Geometry: final body of the model. Coordinates: model frame, mm. A direction names the side the tool comes from. Give positions to 0.01 mm unless a question says otherwise; leave off trailing zeros. Order: outer loops, then holes, each group sorted by start corner. A loop starts at its lowest first (then second) coordinate and runs counter-clockwise, first axis right, second up. Notation, with made-up numbers: (36, -11.5) - (43, -11.5) arc R13 cw to (43, 11.5) - close; hole circle Ø9 at (86, -23.75). An arc over 180 degrees is marked (long way). One line per item, written item: value.
```python
from build123d import *

# Parameters (mm, degrees)
F1_DEPTH  = 6
F2_R      = 1.6
F2_W      = 10
F2_H      = 6
F2_W_2    = 6
F2_H_2    = 10
F3_DEPTH  = 6.001
F4_W      = 6
F4_H      = 10
F5_DEPTH  = 6.001
F7_DEPTH  = 6.001
F8_R      = 10
F9_R      = 8
F9_R_2    = 3
F9_R_3    = 1.5
F10_DEPTH = 6.001
F11_R     = 7.99999


# Not quite as in the source:
# - a fillet or chamfer is up to 0.001 mm smaller than in the source, because OpenCascade refuses the exact size


with BuildPart() as f1:
    # F0 (on Top) → F1 (new body)
    with BuildSketch(Plane.XY):
        Polygon((-150, -150), (150, -150), (150, -20.0961894323), (51.7949192431, 150), (-51.7949192431, 150), (-150, -20.0961894323), align=None)
    extrude(amount=F1_DEPTH)

    # F2 (on face) → F3 (cut, through all)
    with BuildSketch(Plane.XY.offset(6)):
        Polygon((-139.3974596216, -1.7320508076), (-142.3974596216, -6.9282032303), (-133.7372055837, -11.9282032303), (-130.7372055837, -6.7320508076), align=None)
        with Locations((-127.9070785648, -11.8301270189)):
            Circle(F2_R)
        Polygon((-50.7372055837, 131.8320137979), (-59.3974596216, 136.8320137979), (-62.3974596216, 131.6358613752), (-53.7372055837, 126.6358613752), align=None)
        with Locations((-47.9070785648, 126.7339375866)):
            Circle(F2_R)
        Polygon((133.7372055837, -11.9282032303), (142.3974596216, -6.9282032303), (139.3974596216, -1.7320508076), (130.7372055837, -6.7320508076), align=None)
        with Locations((127.9070785648, -11.8301270189)):
            Circle(F2_R)
        Polygon((53.7372055837, 126.6358613752), (62.3974596216, 131.6358613752), (59.3974596216, 136.8320137979), (50.7372055837, 131.8320137979), align=None)
        with Locations((47.9070785648, 126.7339375866)):
            Circle(F2_R)
        with Locations((-145, -35.0480947162)):
            Rectangle(F2_W, F2_H)
        with Locations((-135, -35.0480947162)):
            Circle(F2_R)
        with Locations((-145, -135.0480947162)):
            Rectangle(F2_W, F2_H)
        with Locations((-135, -135.0480947162)):
            Circle(F2_R)
        with Locations((145, -135.0480947162)):
            Rectangle(F2_W, F2_H)
        with Locations((135, -135.0480947162)):
            Circle(F2_R)
        with Locations((135, -35.0480947162)):
            Circle(F2_R)
        with Locations((145, -35.0480947162)):
            Rectangle(F2_W, F2_H)
        with Locations((-35, 145)):
            Rectangle(F2_W_2, F2_H_2)
        with Locations((-35, 135)):
            Circle(F2_R)
        with Locations((35, 145)):
            Rectangle(F2_W_2, F2_H_2)
        with Locations((35, 135)):
            Circle(F2_R)
        with Locations((-100, -145)):
            Rectangle(F2_W_2, F2_H_2)
        with Locations((-100, -135)):
            Circle(F2_R)
        with Locations((100, -135)):
            Circle(F2_R)
        with Locations((100, -145)):
            Rectangle(F2_W_2, F2_H_2)
    extrude(amount=-F3_DEPTH, mode=Mode.SUBTRACT)

    # F4 (on face) → F5 (cut, through all)
    with BuildSketch(Plane.XY.offset(6)):
        with Locations((-11, -145)):
            Rectangle(F4_W, F4_H)
        with Locations((11, -145)):
            Rectangle(F4_W, F4_H)
        Polygon((-107.8397459622, 32.9275126212), (-116.5, 37.9275126212), (-119.5, 32.7313601985), (-110.8397459622, 27.7313601985), align=None)
        Polygon((-105.5, 56.9800715045), (-108.5, 51.7839190818), (-99.8397459622, 46.7839190818), (-96.8397459622, 51.9800715045), align=None)
        Polygon((107.8397459622, 32.9275126212), (110.8397459622, 27.7313601985), (119.5, 32.7313601985), (116.5, 37.9275126212), align=None)
        Polygon((105.5, 56.9800715045), (96.8397459622, 51.9800715045), (99.8397459622, 46.7839190818), (108.5, 51.7839190818), align=None)
    extrude(amount=-F5_DEPTH, mode=Mode.SUBTRACT)

    # F6 (on face) → F7 (cut, through all)
    with BuildSketch(Plane.XY.offset(6)):
        with BuildLine():
            Line((62, -130), (130, -130))
            Line((130, -130), (130, -25.455173281))
            Line((130, -25.455173281), (40.2479138593, 130))
            Line((40.2479138593, 130), (-40.2479138593, 130))
            Line((-40.2479138593, 130), (-130, -25.455173281))
            Line((-130, -25.455173281), (-130, -130))
            Line((-130, -130), (-75, -130))
            Line((-75, -130), (-75, -114))
            Line((-75, -114), (-25, -114))
            Line((-25, -114), (-25, -130))
            Line((-25, -130), (38, -130))
            Line((38, -130), (38, -122))
            ThreePointArc((38, -122), (50, -110), (62, -122))
            Line((62, -122), (62, -130))
        make_face()
    extrude(amount=-F7_DEPTH, mode=Mode.SUBTRACT)

    # F8
    f8_edges = [f1.edges().sort_by_distance(p)[0] for p in [
        (-40.247914, 130, 3),
        (-130, -25.455173, 3),
        (130, -25.455173, 3),
        (40.247914, 130, 3),
        (130, -130, 3),
        (-130, -130, 3),
    ]]
    fillet(f8_edges, radius=F8_R)

    # F9 (on face) → F10 (cut, through all)
    with BuildSketch(Plane.XY.offset(6)):
        with Locations((50, -122)):
            Circle(F9_R)
        with Locations((-67, -122)):
            Circle(F9_R_2)
        with Locations((-57, -122)):
            Circle(F9_R_2)
        with Locations((-39, -122)):
            Circle(F9_R_3)
        with Locations((-33, -122)):
            Circle(F9_R_3)
        with Locations((-45, -122)):
            Circle(F9_R_3)
    extrude(amount=-F10_DEPTH, mode=Mode.SUBTRACT)

    # F11 (radius 8 in the source; OpenCascade refuses exactly that, so slightly less here)
    f11_edges = [f1.edges().sort_by_distance(p)[0] for p in [
        (-75, -130, 3),
        (-75, -114, 3),
        (-25, -114, 3),
        (-25, -130, 3),
        (62, -130, 3),
        (38, -130, 3),
    ]]
    fillet(f11_edges, radius=F11_R)


solid = f1.part
```
1) Section C-C, the plane z = 4.75. Count the separate pieces of the cut face and the enclosed holes in it, then the cut area to 3 significant figures.
Answers below:
separate pieces: 1
enclosed holes: 19
area: 19,500 mm^2
2) First-contact query: pin 1 (3 mm diameter, centred on x = 37, z = 4.5, fed in from +Y); pin 2 (1.8 mm diameter, centred on x = -35, z = 4, fed in from +Y). Flat tips, straight axial feed; report the tip coordinate or a pass-through.
Answers below:
pin 1: y = 150
pin 2: y = 140
3) Mould query, pull axis X, two halves, no side actions, for faces 1 (the face through (-22.594, -127.719, 2.958)), 2 (the face through (84.25, 93.79, 2.96)), 3 (the face through (-1, -133, 0)). Classes: released by +X, released by -X, zero draft, split by the parting line, or undercut.
Answers below:
face 1: undercut
face 2: released by +X
face 3: zero draft
4) Section B-B, the plane y = 83.5. Return loops of the section in (x, z), then the cut area to 3 significant figures.
Answers below:
outline: (-90.19, 0) - (-67.09, 0) - (-67.09, 6) - (-90.19, 6) - close; (67.09, 0) - (90.19, 0) - (90.19, 6) - (67.09, 6) - close
area: 277 mm^2
5) Section A-A, the plane x = -3. Return loops of the section in (y, z).
Answers below:
outline: (-150, 0) - (-130, 0) - (-130, 6) - (-150, 6) - close; (130, 0) - (150, 0) - (150, 6) - (130, 6) - close
6) Set-up query: faces 4 (the face through (-1, -133, 6)), 5 (the face through (-27.281, -116.406, 2.958)). Return all of +Z, -Z, +X, -X, +Y, -Y with unobstructed straight access to the full face (end or side cutting, diameter ignored); none if empty.
Answers below:
face 4: +Z, +X, -X, +Y, -Y
face 5: +Z, -Z
7) Material intervals for line 1 along Y through (x, z) = (-3.5, 0.5); line 2 along X through (y, z) = (135, 3.95), sorted ascending.
Answers below:
line 1: -150 to -130, 130 to 150
line 2: -56.22 to -36.6, -33.4 to 33.4, 36.6 to 56.22
